The model under review builds one solid part; all positions refer to its coordinate system, in mm. Face numbers are marked on the shaded views. A direction names the side the tool comes from. Coordinates: 2 decimals unless noted, no trailing zeros. Write each loop counter-clockwise with the first axis right and the second up, starting at its lowest first coordinate (ties: lowest second). Pieces come first, ordered by that corner, then holes. Notation, with made-up numbers: (64.5, 62.5) -> (74.5, 62.5) arc R16 cw to (74.5, 71.5) -> close; hole circle Ø5 at (29, 60.5). An arc over 180 degrees is marked (long way). Write each question's results on one line, items separated by ' | '.
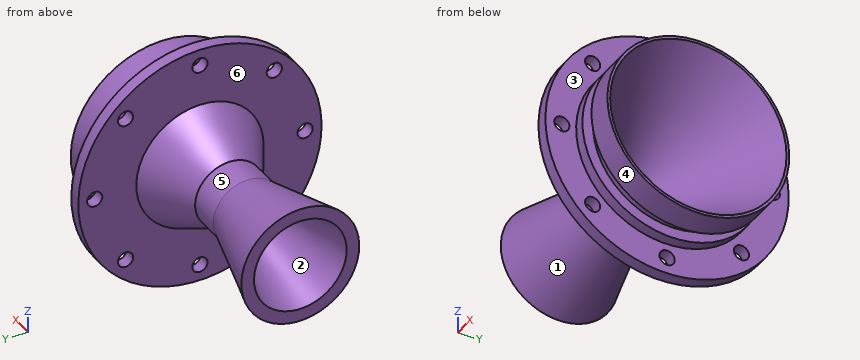
```python
from build123d import *

# Parameters (mm, degrees)
F2_R = 2.54
F5_W = 3.302
F5_H = 4.953003
F8_D = 3.175


with BuildPart() as f1:
    # F0 (on Front) → F1 (revolve)
    with BuildSketch(Plane.XZ):
        Polygon((-23.976779, 4.572), (0, 18.415), (0, 25.4), (-13.97, 25.4), (-13.97, 13.282356), (-24.65737, 7.112), (-31.262382, 7.112), (-50.646779, 12.306034), (-50.646779, 9.676432), (-31.596779, 4.572), align=None)
    revolve(axis=Axis((-17.938589, 0, 0), (-1, 0, 0)))

    # F2
    f2_edges = [f1.edges().sort_by_distance(p)[0] for p in [
        (-23.976779, 0, -4.572),
    ]]
    fillet(f2_edges, radius=F2_R)

    # F3 (on Front) → F4 (revolve, cut)
    with BuildSketch(Plane.XZ):
        Polygon((-11.43, 18.9865), (10.714284, 18.9865), (9.031125, 27.501298), (-11.43, 27.501298), align=None)
    revolve(axis=Axis((6.990795, 0, 0), (1, 0, 0)), mode=Mode.SUBTRACT)

    # F5 (on Front) → F6 (revolve, cut)
    with BuildSketch(Plane.XZ):
        with Locations((-7.493, 19.240502)):
            Rectangle(F5_W, F5_H)
    revolve(axis=Axis((-24.65737, 0, 0), (-1, 0, 0)), mode=Mode.SUBTRACT)

    # F8 (through all)
    with Locations(Plane(origin=(-13.97, 0, 0), x_dir=(0, -1, 0), z_dir=(-1, 0, 0))):
        with Locations((0, 21.971), (15.535843, 15.535843), (21.971, 0), (15.535843, -15.535843), (0, -21.971), (-15.535843, -15.535843), (-21.971, 0), (-15.535843, 15.535843)):
            Hole(F8_D / 2)


solid = f1.part
```
Q1. For line 1 (Y direction, x = -26, z = 0); line 2 (X direction, y = -14, z = 16.5); line 3 (Y direction, x = -45, z = -6.5), list the stretches that pass through material, from the lowest coordinate up. Write a range as from..to.
Solution:
line 1: -7.11..-4.57, 4.57..7.11 | line 2: -13.97..-11.43 | line 3: -8.62..-4.94, 4.94..8.62
Q2. Machinability: for the marked faces 4, 5 and 6, which of the approach directions +Z, -Z, +X, -X, +Y, -Y give a long, thin tool a straight path to every point of the face, cutting with its end or side? Answer none if there is none.
Solution:
face 4: +X | face 5: none | face 6: -X
Q3. Add section D-D (x = -34). Write out the cut boundary in (y, z), plus the area to 3 significant figures.
Solution:
outline: circle Ø15.69 at (0, 0); hole circle Ø10.43 at (0, 0) | area: 108 mm²
Q4. Add section C-C (x = -22.5). Write out the cut boundary in (y, z).
Solution:
outline: circle Ø16.72 at (0, 0); hole circle Ø10.85 at (0, 0)
Q5. Add section A-A (z = 0). Count the separate pieces of the cut face and the enclosed holes in it, plus the area to 3 significant figures.
Solution:
separate pieces: 4 | enclosed holes: 0 | area: 328 mm²
Q6. Clearance check with flat-ended pins moving along their axes: P1, Ø3, axis at y = 15.54, z = 15.54, coming from the -X side; P2, Ø5, axis at x = -31, z = -3, coming from the +Y side; P3, Ø5, axis at y = -21.971, z = 0, coming from the -X side; P4, Ø8, axis at x = -12, z = -9.5, coming from the +Y side. State where each tip first meets the part, or that it passes through.
Solution:
P1: through | P2: y = 7.43 | P3: x = -13.97 | P4: y = 24.8
Q7. Draft analysis for pull direction X (two halves, no side actions). For the marked faces 1, 2 and 3, state which applies: pulls with the +X half, pulls with the -X half, needs draft (parallel to the pull), parting line crosses it, or undercut.
Solution:
face 1: undercut | face 2: pulls with the -X half | face 3: pulls with the +X half
